Source: three-view drawing plus pictorial views. Frame: mm from the lowest corner of the part. A direction names the side the tool comes from. Coordinates: 2 decimals unless noted, no trailing zeros. Write each loop counter-clockwise with the first axis right and the second up, starting at its lowest first coordinate (ties: lowest second). Pieces come first, ordered by that corner, then holes. Notation, with made-up numbers: (-27.75, -2) - (-6.75, -2) arc R22 ccw to (-6.75, 35) - close; hole circle Ø11 at (8.5, 52.5). An arc over 180 degrees is marked (long way). Put each result on its own line as item: value.
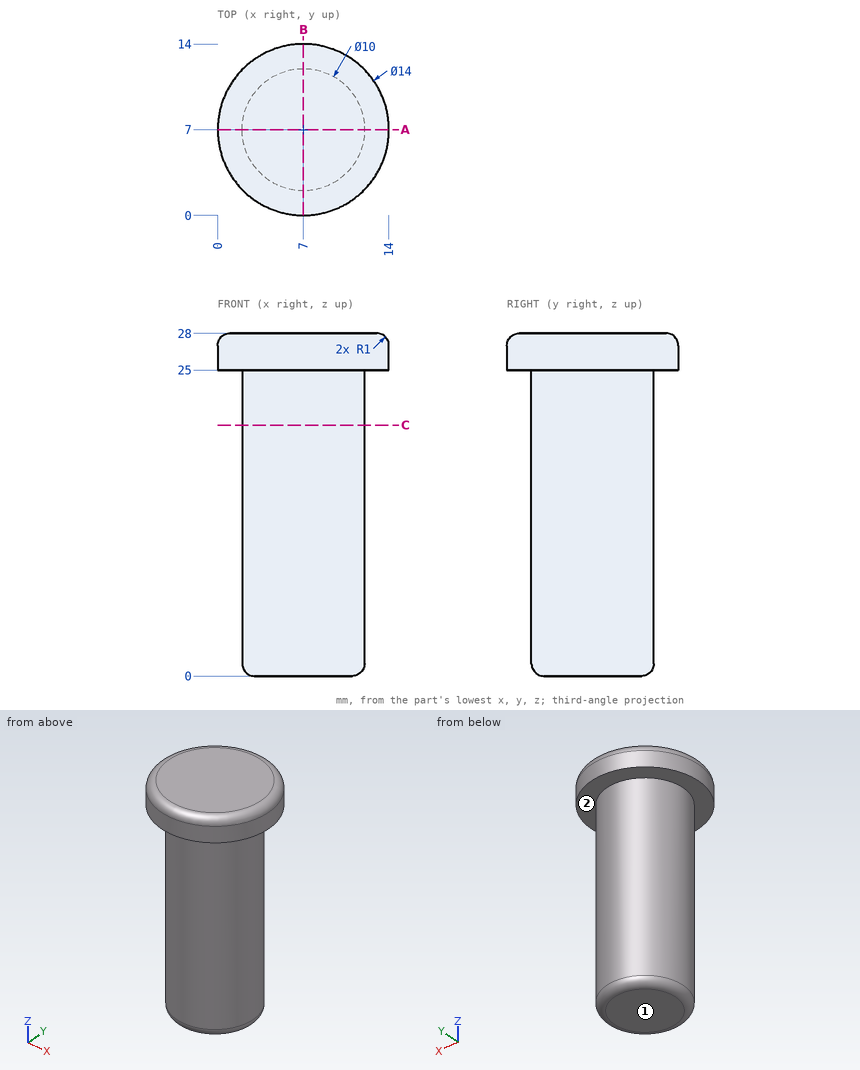
1. Pin query (flat end, axial travel): pin 1 Ø4 at (x, y) = (7.5, 3.5) entering from -Z; pin 2 Ø5 at (x, z) = (8, 13) entering from +Y; pin 3 Ø1 at (y, z) = (1.5, 25) entering from -X; pin 4 Ø8 at (y, z) = (2.5, 9) entering from -X. Return the tip coordinate at first contact, or that it passes through.
Answer below:
pin 1: stops at z = 0
pin 2: stops at y = 12
pin 3: stops at x = 2.1
pin 4: stops at x = 2.03
2. Ray query, probe 1 along Z at (x, y) = (1, 7.5); probe 2 along Y at (x, z) = (7, 6.25); probe 3 along Y at (x, z) = (5.75, 26.5). Return the intervals inside material, ascending. Write a range as from..to.
Answer below:
probe 1: z = 25..28
probe 2: y = 2..12
probe 3: y = 0.11..13.89
3. Section query A-A (y = 7). Return loops of the section in (x, z), then the cut area to 3 significant figures.
Answer below:
outline: (0, 25) - (2, 25) - (2, 1) arc R1 ccw to (3, 0) - (11, 0) arc R1 ccw to (12, 1) - (12, 25) - (14, 25) - (14, 27) arc R1 ccw to (13, 28) - (1, 28) arc R1 ccw to (0, 27) - close
area: 291 mm²
4. Section query C-C (z = 20.5). Return loops of the section in (x, y).
Answer below:
outline: circle Ø10 at (7, 7)
5. Set-up query: the marked faces 1 and 2. Return all of +Z, -Z, +X, -X, +Y, -Y with unobstructed straight access to the full face (end or side cutting, diameter ignored); none if empty.
Answer below:
face 1: -Z, +X, -X, +Y, -Y
face 2: -Z
